from build123d import *

# Parameters (mm, degrees)
F1_DEPTH = 11.1125
F2_R     = 2.15265
F3_DEPTH = 15.875


with BuildPart() as f1:
    # F0 (on Top) → F1 (new body)
    with BuildSketch(Plane.XY):
        with BuildLine():
            Line((-47.625, -15.875), (0, -15.875))
            Line((0, -15.875), (0, 0))
            Line((0, 0), (-11.1125, 0))
            ThreePointArc((-11.1125, 0), (-23.8125, -12.7), (-36.5125, 0))
            Line((-36.5125, 0), (-47.625, 0))
            Line((-47.625, 0), (-47.625, -15.875))
        make_face()
    extrude(amount=F1_DEPTH)

    # F2 (on face) → F3 (cut, through all)
    with BuildSketch(Plane(origin=(0, 0, 0), x_dir=(-1, 0, 0), z_dir=(0, 1, 0))):
        with Locations((43.65625, 5.55625)):
            Circle(F2_R)
        with Locations((3.96875, 5.55625)):
            Circle(F2_R)
    extrude(amount=-F3_DEPTH, mode=Mode.SUBTRACT)


solid = f1.part
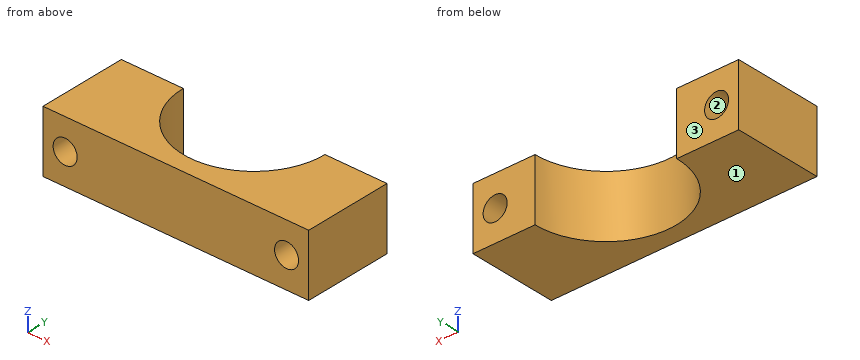
For this review, take the finished solid that the model builds, in its own axes (mm). Face numbers are marked on the shaded views. Round coordinates to 2 decimals unless told otherwise and drop trailing zeros. Order: outer loops, then holes, each group sorted by start corner. A loop starts at its lowest first (then second) coordinate and runs counter-clockwise, first axis right, second up. Notation, with made-up numbers: M -12.75,15 L 2.25,15 A22 cw 2.25,38 Z; hole C -14,16 d2. An arc over 180 degrees is marked long. Use a Markdown table: item, result. Add a question column.
Item 1: Add section D-D, the plane z = 8.75. Give the boundary of the cut face in (x, y) (1 decimal).
Item 2: Insertion check: pin 1 (2 mm diameter, centred on x = -29.5, y = -9, fed in from -Z). The pin has a flat end and moves straight along its axis. Give the tip position at first contact, or say it passes through.
Item 3: Add section A-A, the plane y = -9. Give the boundary of the cut face in (x, z) (1 decimal), then the cut area to 3 significant figures.
Item 4: Add section C-C, the plane z = 6. Give the boundary of the cut face in (x, y) (1 decimal).
Item 5: Add section B-B, the plane x = -4.5. Give the boundary of the cut face in (y, z) (1 decimal), then the cut area to 3 significant figures.
Item 6: To check wall thickness, follow line 1 along X through (y, z) = (-3, 7) (3 decimals); line 2 along X through (y, z) = (-8.5, 9.5) (3 decimals); line 3 along X through (y, z) = (-3, 2.5) (3 decimals). State the ranges of each line that lie inside material, in increasing order.
Item 7: Mouldability with a two-part tool opening along Z and no side actions: class the marked faces 1, 2 and 3 as released by +Z, released by -Z, zero draft, split by the parting line, or undercut.
Geometry results:
| question | item | result |
|---|---|---|
| 1 | outline | M -47.6,-15.9 L 0,-15.9 L 0,0 L -11.1,0 A12.7 cw -36.5,0 L -47.6,0 Z |
| 2 | pin 1 | passes through |
| 3 | outline | M -47.6,0 L -32.8,0 L -32.8,11.1 L -47.6,11.1 Z; M -14.9,0 L 0,0 L 0,11.1 L -14.9,11.1 Z; hole C -43.7,5.6 d4.3; hole C -4,5.6 d4.3 |
| 3 | area | 301 mm² |
| 4 | outline | M -47.6,-15.9 L -45.8,-15.9 L -45.8,0 L -47.6,0 Z; M -41.5,-15.9 L -6.1,-15.9 L -6.1,0 L -11.1,0 A12.7 cw -36.5,0 L -41.5,0 Z; M -1.9,-15.9 L 0,-15.9 L 0,0 L -1.9,0 Z |
| 5 | outline | M -15.9,0 L 0,0 L 0,3.5 L -15.9,3.5 Z; M -15.9,7.6 L 0,7.6 L 0,11.1 L -15.9,11.1 Z |
| 5 | area | 110 mm² |
| 6 | line 1 | x = -47.625 to -45.253, -42.06 to -36.153, -11.472 to -5.565, -2.372 to 0 |
| 6 | line 2 | x = -47.625 to -33.249, -14.376 to 0 |
| 6 | line 3 | x = -47.625 to -36.153, -11.472 to 0 |
| 7 | face 1 | released by -Z |
| 7 | face 2 | undercut |
| 7 | face 3 | zero draft |
